from build123d import *

# Parameters (mm, degrees)
CROQUIS1_R              = 107.5
SALIENTE_EXTRUIR1_DEPTH = 10
MATRIZC1_COUNT          = 6
CROQUIS4_R              = 55
CORTAR_EXTRUIR1_DEPTH   = 10


with BuildPart() as part:
    # Croquis1 → Saliente-Extruir1 (new body)
    with BuildSketch(Plane(origin=(0, 0, 0), x_dir=(1, 0, 0), z_dir=(0, 1, 0))):
        with Locations(Location((0, 0, 0), (0, 0, 270))):
            Circle(CROQUIS1_R)
    extrude(amount=SALIENTE_EXTRUIR1_DEPTH)

    # Croquis6 → Taladro roscado M12x1.51 (revolve, cut)
    with BuildSketch(Plane(origin=(0, 10, -97.5), x_dir=(0, 0, 1), z_dir=(1, 0, 0))):
        Polygon((0, 0), (0, 34.65451825), (5.25, 31.5), (5.25, 0), align=None)
    taladro_roscado_m12x1_51 = revolve(axis=Axis((0, 16.35, -97.5), (0, -1, 0)), mode=Mode.SUBTRACT)

    # MatrizC1: Taladro roscado M12x1.51 ×6 about axis
    matrizc1_axis = Axis((0, 0, 0.233100581), (0, 1, 0))
    for i in range(1, MATRIZC1_COUNT):
        add(taladro_roscado_m12x1_51.rotate(matrizc1_axis, i * 360 / MATRIZC1_COUNT), mode=Mode.SUBTRACT)

    # Croquis4 → Cortar-Extruir1 (cut)
    with BuildSketch(Plane(origin=(0, 10, 0), x_dir=(1, 0, 0), z_dir=(0, 1, 0))):
        with Locations(Location((0, 0, 0), (0, 0, 270))):
            Circle(CROQUIS4_R)
    extrude(amount=-CORTAR_EXTRUIR1_DEPTH, mode=Mode.SUBTRACT)


solid = part.part
Can you work these out from the model? Positions are in its coordinate system, mm. Round coordinates to 2 decimals unless told otherwise and drop trailing zeros. Order: outer loops, then holes, each group sorted by start corner. A loop starts at its lowest first (then second) coordinate and runs counter-clockwise, first axis right, second up. Notation, with made-up numbers: M 69.5,34 L 84.5,34 A24 cw 84.5,52 Z; hole C 27,-16 d5. An arc over 180 degrees is marked long. Use a Markdown table: item, result.
1) I'm going to push flat-ended pins straight in: P1, Ø5, axis at x = -83.5, y = 2, coming from the -Z side; P2, Ø5, axis at x = 64, y = 2.5, coming from the -Z side; P3, Ø1.5, axis at y = 3.5, z = -13, coming from the -X side. Where does each tip first touch, or does it pass through?
Geometry says:
| item | result |
|---|---|
| P1 | stops at z = -70.68 |
| P2 | stops at z = -88.17 |
| P3 | stops at x = -106.8 |
2) Imagine slicing it at D-D (x = -42.5). List the corners of the cut face in (y, z) for me.
Geometry says:
| item | result |
|---|---|
| outline | M 0,-98.74 L 10,-98.74 L 10,-34.91 L 0,-34.91 Z; M 0,34.91 L 10,34.91 L 10,98.74 L 0,98.74 Z |
3) Imagine slicing it at B-B (x = 0). List the corners of the cut face in (y, z) for me, then the cut area to 3 significant figures.
Geometry says:
| item | result |
|---|---|
| outline | M 0,-107.5 L 10,-107.5 L 10,-102.75 L 0,-102.75 Z; M 0,-92.25 L 10,-92.25 L 10,-55 L 0,-55 Z; M 0,55 L 10,55 L 10,92.72 L 0,92.72 Z; M 0,103.22 L 10,103.22 L 10,107.5 L 0,107.5 Z |
| area | 840 mm² |
4) Imagine slicing it at A-A (z = 0). List the corners of the cut face in (x, y) for me.
Geometry says:
| item | result |
|---|---|
| outline | M -107.5,0 L -55,0 L -55,10 L -107.5,10 Z; M 55,0 L 107.5,0 L 107.5,10 L 55,10 Z |
5) Imagine slicing it at C-C (y = 4). List the corners of the cut face in (x, z) for me.
Geometry says:
| item | result |
|---|---|
| outline | C 0,0 d215; hole C -84.64,-48.63 d10.5; hole C -84.64,49.1 d10.5; hole C 0,0 d110; hole C 0,-97.5 d10.5; hole C 0,97.97 d10.5; hole C 84.64,-48.63 d10.5; hole C 84.64,49.1 d10.5 |
6) If we mould it in two halves opening along Z, with no side actions, what happens to faces 1 (the face through (-1.6, 5.1, -92.5)), 2 (the face through (0.23, 5.07, 103.21)), 3 (the face through (-104.944, 4.93, -23.304)), 4 (the face through (25.4, 0, -49.3))? For each: +Z half, -Z half, draft (parallel to the pull), parting line (faces both ways), or undercut.
Geometry says:
| item | result |
|---|---|
| face 1 | undercut |
| face 2 | undercut |
| face 3 | parting line |
| face 4 | draft |
7) If I drill on line 1 along X through (y, z) = (4.75, 48); line 2 along Z through (x, y) = (3, 5.75); line 3 along X through (y, z) = (3.5, -50.5), over which ranges is the centre line in solid material (lowest first)?
Geometry says:
| item | result |
|---|---|
| line 1 | x = -96.19 to -89.77, -79.51 to -26.85, 26.85 to 79.51, 89.77 to 96.19 |
| line 2 | z = -107.46 to -101.81, -93.19 to -54.92, 54.92 to 93.66, 102.27 to 107.46 |
| line 3 | x = -94.9 to -89.55, -79.73 to -21.79, 21.79 to 79.73, 89.55 to 94.9 |
